Work out the finished part from the listing and answer in its coordinate system (mm). Face numbers are marked on the shaded views. A direction names the side the tool comes from. Coordinates: 2 decimals unless noted, no trailing zeros. Write each loop counter-clockwise with the first axis right and the second up, starting at its lowest first coordinate (ties: lowest second). Pieces come first, ordered by that corner, then holes. Notation, with made-up numbers: M -17.75,18 L 18.25,18 A13 cw 18.25,25 Z; hole C -23,-20.5 d6. An arc over 180 degrees is marked long. Answer as CSV lines item,"result". Start each with the question number.
(1) A cutting plane is placed at C-C on z = 20. Give the vertices of the cut face in (x, y), then the cut area to 3 significant figures.
(2) A cutting plane is placed at B-B on x = 6. Give the vertices of the cut face in (y, z), then the cut area to 3 significant figures.
(3) A cutting plane is placed at D-D on x = 19. Give the vertices of the cut face in (y, z), then the cut area to 3 significant figures.
(4) For the marked faces 1, 2 and 3, determine the directions among +Z, -Z, +X, -X, +Y, -Y from which every point of the face is accessible in a straight line to the end or side of a thin tool.
(5) A cutting plane is placed at A-A on y = 22. Give the vertices of the cut face in (x, z).
(6) Flat-ended cylindrical pins translate along their axes: P1, Ø6.5, axis at x = 37.5, z = 9, coming from the -Y side; P2, Ø1.7, axis at x = 21, z = 27.5, coming from the +Y side; P3, Ø3, axis at x = 42.5, z = 25.5, coming from the +Y side. Find the tip coordinate at first contact, or state that the pin passes through.
(7) Find the intervals of material crossed by L1, parallel to X at y = 28.75, z = 20; L2, parallel to Z at x = 32.5, y = 22; L3, parallel to X at y = 27, z = 17.5, in increasing order. Write a range as [from, to].
from build123d import *

# Parameters (mm, degrees)
BOSS_EXTRUDE3_DEPTH = 40
SKETCH7_W           = 14
SKETCH7_H           = 14
CUT_EXTRUDE3_DEPTH  = 108
SKETCH8_R           = 4
CUT_EXTRUDE4_DEPTH  = 108
SKETCH9_W           = 24
SKETCH9_H           = 24
CUT_EXTRUDE5_DEPTH  = 8
SKETCH10_R          = 9
CUT_EXTRUDE6_DEPTH  = 9
SKETCH11_R          = 9
CUT_EXTRUDE7_DEPTH  = 9


with BuildPart() as part:
    # Sketch1 → Boss-Extrude3 (new body)
    with BuildSketch(Plane.XY):
        Polygon((10, 0), (10, 8), (60, 8), (60, 0), (70, 0), (70, 41), (0, 41), (0, 0), align=None)
    extrude(amount=BOSS_EXTRUDE3_DEPTH)

    # Sketch7 → Cut-Extrude3 (cut)
    with BuildSketch(Plane(origin=(70, 0, 0), x_dir=(0, 0, -1), z_dir=(1, 0, 0))):
        with Locations((-20, 7)):
            Rectangle(SKETCH7_W, SKETCH7_H)
    extrude(amount=-CUT_EXTRUDE3_DEPTH, mode=Mode.SUBTRACT)

    # Sketch8 → Cut-Extrude4 (cut)
    with BuildSketch(Plane(origin=(70, 0, 0), x_dir=(0, 0, -1), z_dir=(1, 0, 0))):
        with Locations(Location((-20, 22, 0), (0, 0, 90))):
            Circle(SKETCH8_R)
    extrude(amount=-CUT_EXTRUDE4_DEPTH, mode=Mode.SUBTRACT)

    # Sketch9 → Cut-Extrude5 (cut)
    with BuildSketch(Plane(origin=(0, 41, 0), x_dir=(1, 0, 0), z_dir=(0, 1, 0))):
        with Locations((19, -20)):
            Rectangle(SKETCH9_W, SKETCH9_H)
        with Locations((51, -20)):
            Rectangle(SKETCH9_W, SKETCH9_H)
    extrude(amount=-CUT_EXTRUDE5_DEPTH, mode=Mode.SUBTRACT)

    # Sketch10 → Cut-Extrude6 (cut)
    with BuildSketch(Plane(origin=(0, 33, 0), x_dir=(1, 0, 0), z_dir=(0, 1, 0))):
        with Locations(Location((19, -20, 0), (0, 0, 270))):
            Circle(SKETCH10_R)
    extrude(amount=-CUT_EXTRUDE6_DEPTH, mode=Mode.SUBTRACT)

    # Sketch11 → Cut-Extrude7 (cut)
    with BuildSketch(Plane(origin=(0, 33, 0), x_dir=(1, 0, 0), z_dir=(0, 1, 0))):
        with Locations(Location((51, -20, 0), (0, 0, 270))):
            Circle(SKETCH11_R)
    extrude(amount=-CUT_EXTRUDE7_DEPTH, mode=Mode.SUBTRACT)


solid = part.part
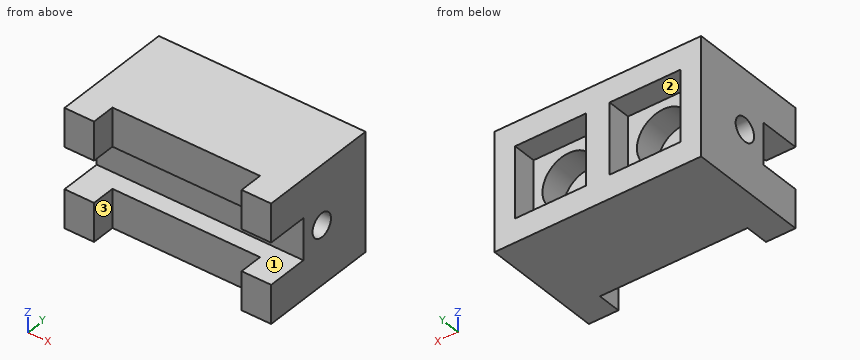
Here are the results:
1,outline,"M 0,14 L 70,14 L 70,18 L 0,18 Z; M 0,26 L 10,26 L 10,33 L 7,33 L 7,41 L 0,41 Z; M 28,26 L 42,26 L 42,33 L 39,33 L 39,41 L 31,41 L 31,33 L 28,33 Z; M 60,26 L 70,26 L 70,41 L 63,41 L 63,33 L 60,33 Z"
1,area,"694 mm^2"
2,outline,"M 0,0 L 41,0 L 41,40 L 0,40 L 0,27 L 14,27 L 14,13 L 0,13 Z; hole C 22,20 d8"
2,area,"1,390 mm^2"
3,outline,"M 8,0 L 41,0 L 41,8 L 33,8 L 33,11 L 24,11 L 24,16.54 A4 cw long 24,23.46 L 24,29 L 33,29 L 33,32 L 41,32 L 41,40 L 8,40 L 8,27 L 14,27 L 14,13 L 8,13 Z"
3,area,"842 mm^2"
4,face 1,"+X, -X, -Y"
4,face 2,"+Y"
4,face 3,"+Z, -Z, -Y"
5,outline,"M 0,0 L 70,0 L 70,16 L 0,16 Z; M 0,24 L 70,24 L 70,40 L 0,40 Z"
6,P1,"stops at y = 8"
6,P2,"stops at y = 24"
6,P3,"stops at y = 33"
7,L1,"x = [0, 10], [28, 42], [60, 70]"
7,L2,"z = [0, 16], [24, 40]"
7,L3,"x = [0, 10.35], [27.65, 42.35], [59.65, 70]"
